```python
from build123d import *

# Parameters (mm, degrees)
SKETCH_1_R      = 2
EXTRUDE_1_DEPTH = 2.2
CHAMFER_1_SIZE  = 0.3


with BuildPart() as part:
    # Эскиз1 → Бобышка-Вытянуть1 (new body)
    with BuildSketch(Plane(origin=(0, 0, 0), x_dir=(1, 0, 0), z_dir=(0, 1, 0))):
        Polygon((-3.5, 2.020725942), (-3.5, -2.020725942), (0, -4.041451884), (3.5, -2.020725942), (3.5, 2.020725942), (0, 4.041451884), align=None)
        Circle(SKETCH_1_R, mode=Mode.SUBTRACT)
    extrude(amount=EXTRUDE_1_DEPTH)

    # Фаска1
    chamfer_1_edges = [part.edges().sort_by_distance(p)[0] for p in [
        (-2, 0, 0),
        (-2, 2.2, 0),
    ]]
    chamfer(chamfer_1_edges, length=CHAMFER_1_SIZE)


solid = part.part
```
The listing builds one solid part. Answer for the finished solid, in the listing's coordinates (mm). Coordinates: 2 decimals unless noted, no trailing zeros. Write each loop counter-clockwise with the first axis right and the second up, starting at its lowest first coordinate (ties: lowest second). Pieces come first, ordered by that corner, then holes. Notation, with made-up numbers: M -29,35.25 L -4,35.25 A17 ccw -4,59.25 Z; hole C 22.25,54.5 d11. An arc over 180 degrees is marked long. Use a Markdown table: item, result. Add a question column.
1. Straight lines are drawn through the part: line 1 along X through (y, z) = (1.1, 0); line 2 along Z through (x, y) = (-0.5, 2); line 3 along X through (y, z) = (1.55, -1.25). For each, find the intervals that lie inside material, in ascending order. Write a range as [from, to].
2. For a pull along X with two mould halves and no side action, classify faces 1 (the flat face through (-2, 0, 2)), 2 (the cylindrical face through (0, 1, 2)), 3 (the flat face through (-3.5, 1, 0)), 4 (the flat face through (1.8, 1.1, -3)) as +X half, -X half, draft (parallel to the pull), parting line (faces both ways), or undercut.
3. Given P1, Ø1, axis at x = -2.5, y = 1, coming from the -Z side, flat-ended and moving along its own axis, determine where the tip first touches the part or whether it passes through.
4. Section C-C (x = 2.5) is taken. Give the vertices of the cut face in (y, z), plus the area to 3 significant figures.
5. Section A-A (z = 0) is taken. Give the vertices of the cut face in (x, y), plus the area to 3 significant figures.
6. Section D-D (z = 3) is taken. Give the vertices of the cut face in (x, y), plus the area to 3 significant figures.
7. Section B-B (y = 2) is taken. Give the vertices of the cut face in (x, z), plus the area to 3 significant figures.
Data:
| question | item | result |
|---|---|---|
| 1 | line 1 | x = [-3.5, -2], [2, 3.5] |
| 1 | line 2 | z = [-3.75, -2.04], [2.04, 3.75] |
| 1 | line 3 | x = [-3.5, -1.56], [1.56, 3.5] |
| 2 | face 1 | draft |
| 2 | face 2 | undercut |
| 2 | face 3 | -X half |
| 2 | face 4 | +X half |
| 3 | P1 | stops at z = -2.89 |
| 4 | outline | M 0,-2.6 L 2.2,-2.6 L 2.2,2.6 L 0,2.6 Z |
| 4 | area | 11.4 mm2 |
| 5 | outline | M -3.5,0 L -2.3,0 L -2,0.3 L -2,1.9 L -2.3,2.2 L -3.5,2.2 Z; M 2,0.3 L 2.3,0 L 3.5,0 L 3.5,2.2 L 2.3,2.2 L 2,1.9 Z |
| 5 | area | 6.42 mm2 |
| 6 | outline | M -1.8,0 L 1.8,0 L 1.8,2.2 L -1.8,2.2 Z |
| 6 | area | 7.94 mm2 |
| 7 | outline | M -3.5,-2.02 L 0,-4.04 L 3.5,-2.02 L 3.5,2.02 L 0,4.04 L -3.5,2.02 Z; hole C 0,0 d4.2 |
| 7 | area | 28.6 mm2 |
